CAD build for the part. Positions are in the model's coordinates, mm. A direction names the side the tool comes from. Give positions to 0.01 mm unless a question says otherwise; leave off trailing zeros. Order: outer loops, then holes, each group sorted by start corner. A loop starts at its lowest first (then second) coordinate and runs counter-clockwise, first axis right, second up. Notation, with made-up numbers: (70, 55.25) -> (98, 55.25) arc R23 ccw to (98, 63.25) -> close; hole circle Ø9 at (-33, -28.5). An arc over 180 degrees is marked (long way). Use one line per item in the form item = value. Start each with the question number.
1) Cut at D-D, the plane x = -15. Give the cut face in (y, z).
2) Probe line 1 (Y direction, x = -25.5, z = 22.5); line 2 (Z direction, x = 22, y = -40.5); line 3 (Z direction, x = -10, y = -22). List the from-to ranges inside material, lowest first.
3) Cut at A-A, the plane y = -29. Give the cut face in (x, z).
4) Drop flat-ended pins along their axis: P1, Ø9.5, axis at x = 26, z = 15.5, coming from the -Y side; P2, Ø3, axis at y = -15.5, z = 7, coming from the +X side; P3, Ø19, axis at x = 28, y = -47, coming from the +Z side. Give the stop position or say it passes through.
5) Tool access for faces 1 (the face through (58.965, -31, -16)), 2 (the face through (36, -44, 0)), 3 (the face through (-36, -44, 0)): list every direction of +Z, -Z, +X, -X, +Y, -Y with a clear straight run to the whole face (end or side of a thin tool).
6) Cut at C-C, the plane z = 9. Give the cut face in (x, y), and give its area (3 significant figures).
7) Cut at B-B, the plane x = 7. Give the cut face in (y, z).
from build123d import *

# Parameters (mm, degrees)
F0_W     = 117.9294288158
F0_H     = 31.6627249122
F1_DEPTH = 63.5
F2_DEPTH = 25.4
F3_W     = 27.4915890768
F3_H     = 38.1
F4_DEPTH = 31.75
F6_DEPTH = 73.1855023111


with BuildPart() as f1:
    # F0 (on Front) → F1 (new body)
    with BuildSketch(Plane.XZ):
        with Locations((0, -15.8313624561)):
            Rectangle(F0_W, F0_H)
    extrude(amount=F1_DEPTH)

    # F0 (on Front) → F2 (join)
    with BuildSketch(Plane.XZ):
        Polygon((58.9647144079, 0), (23.699644953, 31.6627249122), (-58.9647144079, 31.6627249122), (-58.9647144079, 0), align=None)
    extrude(amount=F2_DEPTH)

    # F3 (on face) → F4 (join)
    with BuildSketch(Plane.XY):
        with Locations((0.4739933647, -44.45)):
            Rectangle(F3_W, F3_H)
    extrude(amount=F4_DEPTH)

    # F5 (on face) → F6 (cut, through all)
    with BuildSketch(Plane.YZ.offset(14.2197879031)):
        Polygon((-63.5, 0), (-25.4, 31.75), (-63.5, 31.75), align=None)
    extrude(amount=-F6_DEPTH, mode=Mode.SUBTRACT)


solid = f1.part
Result:
q1.outline = (-63.5, -31.66) -> (0, -31.66) -> (0, 31.66) -> (-25.4, 31.66) -> (-25.4, 0) -> (-63.5, 0) -> close
q2.line_1 = -25.4 to 0
q2.line_2 = -31.66 to 0
q2.line_3 = -31.66 to 31.66
q3.outline = (-58.96, -31.66) -> (58.96, -31.66) -> (58.96, 0) -> (14.22, 0) -> (14.22, 28.75) -> (-13.27, 28.75) -> (-13.27, 0) -> (-58.96, 0) -> close
q4.P1 = -25.4
q4.P2 = 52.84
q4.P3 = 0
q5.face_1 = +Z, -Z, +X, +Y, -Y
q5.face_2 = +Z, +X, -Y
q5.face_3 = +Z, -X, -Y
q6.outline = (-58.96, -25.4) -> (-13.27, -25.4) -> (-13.27, -52.7) -> (14.22, -52.7) -> (14.22, -25.4) -> (48.94, -25.4) -> (48.94, 0) -> (-58.96, 0) -> close
q6.area = 3,490 mm²
q7.outline = (-63.5, -31.66) -> (0, -31.66) -> (0, 31.66) -> (-25.4, 31.66) -> (-25.4, 31.75) -> (-63.5, 0) -> close
